from build123d import *

# Parameters (mm, degrees)
F1_DEPTH = 5


with BuildPart() as f1:
    # F0 (on Top) → F1 (new body)
    with BuildSketch(Plane.XY):
        with BuildLine():
            ThreePointArc((5.090661, 2.673513), (0, -5.75), (-5.090661, 2.673513))
            ThreePointArc((-5.090661, 2.673513), (-5.071855, 2.859275), (-5.186994, 3.006259))
            Line((-5.186994, 3.006259), (-6.706691, 3.883657))
            ThreePointArc((-6.706691, 3.883657), (-7.48463, 2.010677), (-7.75, 0))
            ThreePointArc((-7.75, 0), (-5.480078, -5.480078), (0, -7.75))
            ThreePointArc((0, -7.75), (5.480078, -5.480078), (7.75, 0))
            ThreePointArc((7.75, 0), (7.48463, 2.010677), (6.706691, 3.883657))
            Line((6.706691, 3.883657), (5.186994, 3.006259))
            ThreePointArc((5.186994, 3.006259), (5.071855, 2.859275), (5.090661, 2.673513))
        make_face()
        with BuildLine():
            ThreePointArc((0, -7.75), (-5.480078, -5.480078), (-7.75, 0))
            Line((-7.75, 0), (-7.75, -5.75))
            ThreePointArc((-7.75, -5.75), (-7.164214, -7.164214), (-5.75, -7.75))
            Line((-5.75, -7.75), (0, -7.75))
        make_face()
        with BuildLine():
            Line((7.75, -5.75), (7.75, 0))
            ThreePointArc((7.75, 0), (5.480078, -5.480078), (0, -7.75))
            Line((0, -7.75), (5.75, -7.75))
            ThreePointArc((5.75, -7.75), (7.164214, -7.164214), (7.75, -5.75))
        make_face()
    extrude(amount=F1_DEPTH)


solid = f1.part
CAD build for the part. Positions are in the model's coordinates, mm. A direction names the side the tool comes from. Round coordinates to 2 decimals unless told otherwise and drop trailing zeros. Loops run counter-clockwise (first coordinate to the right, second up) from the corner with the lowest first, then second, coordinate; pieces in that order, holes last.
(1) Two-plate mould, pull along X, no slides. Class faces 1 (the cylindrical face through (-7.477, 2.038, 2.465)), 2 (the flat face through (0, -7.75, 2)), 3 (the cylindrical face through (0.165, -5.748, 2.465)), 4 (the flat face through (-5.94, 3.44, 2.46)): +X half, -X half, draft (parallel to the pull), parting line (faces both ways), or undercut.
(2) Cut at B-B (x = 0). Give the cut face in (y, z).
(3) Wall check: line 1 along Y through (x, z) = (0, 3.6); line 2 along X through (y, z) = (2, 2.55); line 3 along X through (y, z) = (2.25, 2.7). Give the ranges that are in metal, low to high.
(4) Which spindle directions (+Z, -Z, +X, -X, +Y, -Y) get a long thin tool onto all of the face, cutting with end or side? Do faces 5 (the flat face through (7.75, -3, 2)), 6 (the flat face through (5.957, 3.451, 2.465)). Say none if no direction does.
(5) Cut at A-A (y = -3.25). Give the cut face in (x, z), plus the area to 3 significant figures.
(6) Cut at C-C (z = 4.2). Give the cut face in (x, y), plus the area to 3 significant figures.
(7) Cut at D-D (y = -2). Give the cut face in (x, z).
Findings below:
1. face 1: -X half
1. face 2: draft
1. face 3: undercut
1. face 4: undercut
2. outline: (-7.75, 0) - (-5.75, 0) - (-5.75, 5) - (-7.75, 5) - close
3. line 1: y = -7.75 to -5.75
3. line 2: x = -7.49 to -5.39, 5.39 to 7.49
3. line 3: x = -7.42 to -5.29, 5.29 to 7.42
4. face 5: +Z, -Z, +X, +Y, -Y
4. face 6: +Z, -Z, +Y
5. outline: (-7.75, 0) - (-4.74, 0) - (-4.74, 5) - (-7.75, 5) - close; (4.74, 0) - (7.75, 0) - (7.75, 5) - (4.74, 5) - close
5. area: 30.1 mm2
6. outline: (-7.75, -5.75) arc R2 ccw to (-5.75, -7.75) - (5.75, -7.75) arc R2 ccw to (7.75, -5.75) - (7.75, 0) arc R7.75 ccw to (6.71, 3.88) - (5.19, 3.01) arc R0.25 ccw to (5.09, 2.67) arc R5.75 cw (long way) to (-5.09, 2.67) arc R0.25 ccw to (-5.19, 3.01) - (-6.71, 3.88) arc R7.75 ccw to (-7.75, 0) - close
6. area: 80.6 mm2
7. outline: (-7.75, 0) - (-5.39, 0) - (-5.39, 5) - (-7.75, 5) - close; (5.39, 0) - (7.75, 0) - (7.75, 5) - (5.39, 5) - close
